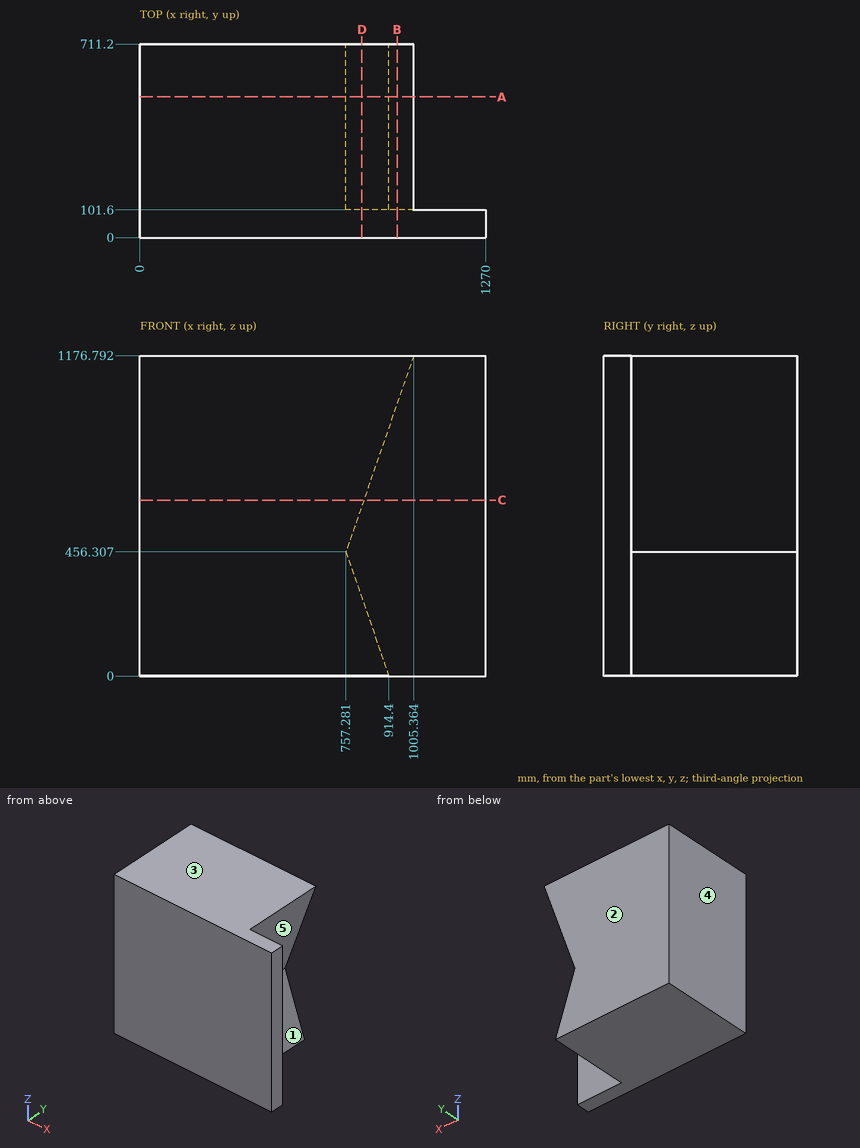
Input: dimensioned drawing with shaded views. Units: mm. Origin: part minimum x, y, z. A direction names the side the tool comes from. Coordinates: 2 decimals unless noted, no trailing zeros. Write each loop counter-clockwise with the first axis right and the second up, starting at its lowest first coordinate (ties: lowest second). Pieces come first, ordered by that corner, then holes. Notation, with made-up numbers: M -21,11 L 14,11 A22 cw 14,26 Z; hole C -21.5,41 d5. An arc over 180 degrees is marked long. Answer as a JSON object with one key per item and string values. Group by question number.
(1) Section B-B on x = 945. Output: boundary loops of the cut face in (y, z), plus the area to 3 significant figures.
(2) Section D-D on x = 816. Output: boundary loops of the cut face in (y, z) (1 decimal).
(3) Section A-A on y = 517. Output: boundary loops of the cut face in (x, z), plus the area to 3 significant figures.
(4) Set-up query: the marked faces 4 and 5. Return all of +Z, -Z, +X, -X, +Y, -Y with unobstructed straight access to the full face (end or side cutting, diameter ignored); none if empty.
(5) Ray query, line 1 along Y through (x, z) = (1016, 376); line 2 along X through (y, z) = (538.5, 520.5) (1 decimal); line 3 along X through (y, z) = (506, 905.5). Return the intervals inside material, ascending. Write a range as [from, to].
(6) Mould query, pull axis Z, two halves, no side actions, for the marked faces 1, 2 and 3. Classes: pulls with the +Z half, pulls with the -Z half, needs draft (parallel to the pull), parting line crosses it, or undercut.
(7) Section C-C on z = 646. Output: boundary loops of the cut face in (x, y).
(8) Contact query for a flat-ended pin moving along its axis: P1, Ø2, axis at x = 866.5, z = 287, coming from the +Y side. Output: stop coordinate, or through.
Result set:
{
 "1": {"outline": "M 0,0 L 101.6,0 L 101.6,1001.48 L 711.2,1001.48 L 711.2,1176.79 L 0,1176.79 Z", "area": "226,000 mm2"},
 "2": {"outline": "M 0,0 L 711.2,0 L 711.2,285.8 L 101.6,285.8 L 101.6,626.8 L 711.2,626.8 L 711.2,1176.8 L 0,1176.8 Z"},
 "3": {"outline": "M 0,0 L 914.4,0 L 757.28,456.31 L 1005.36,1176.79 L 0,1176.79 Z", "area": "1,020,000 mm2"},
 "4": {"face 4": "+Z, -Z, -X, +Y, -Y", "face 5": "+X, +Y"},
 "5": {"line 1": "y = [0, 101.6]", "line 2": "x = [0, 779.4]", "line 3": "x = [0, 911.95]"},
 "6": {"face 1": "undercut", "face 2": "needs draft", "face 3": "pulls with the +Z half"},
 "7": {"outline": "M 0,0 L 1270,0 L 1270,101.6 L 822.6,101.6 L 822.6,711.2 L 0,711.2 Z"},
 "8": {"P1": "stops at y = 101.6"}
}
